```python
from build123d import *

# Parameters (mm, degrees)
BASE_FLANGE1_DEPTH     = 1
SKETCHED_START         = -30
SKETCHED_BEND5_DEPTH   = 60
SKETCHED_BEND5_2_DEPTH = 15
SKETCHED_START_2       = 15
SKETCHED_BEND5_3_DEPTH = 15
SKETCHED_BEND5_4_DEPTH = 60
SKETCHED_START_3       = -15
SKETCHED_BEND5_5_DEPTH = 30
SKETCHED_BEND6_DEPTH   = 60
SKETCHED_BEND6_2_DEPTH = 15
SKETCHED_BEND6_3_DEPTH = 15
SKETCHED_BEND6_4_DEPTH = 30
SKETCHED_BEND6_5_DEPTH = 60
SKETCHED_START_4       = -28.356310605
SKETCHED_BEND7_DEPTH   = 23
SKETCHED_BEND7_2_DEPTH = 23
SKETCHED_START_5       = 11.547743288
SKETCHED_BEND8_DEPTH   = 70
SKETCHED_BEND8_2_DEPTH = 70
SKETCH36_W             = 19.9
SKETCH36_H             = 40.84
CUT_EXTRUDE1_DEPTH     = 10
F_6_CLEARANCE_HOLE4_D  = 3.7973
F_6_CLEARANCE_HOLE2_D  = 3.7973
M1_6_CLEARANCE_HOLE1_D = 1.8
FILLET2_R              = 13
F_2_CLEARANCE_HOLE1_D  = 2.4384
CUT_EXTRUDE2_DEPTH     = 10
FILLET1_R              = 1


# Read off the part's stored shape, not the designer's step: Sketched Bend5, Sketched Bend6, Sketched Bend7, Sketched Bend8
# Sheet-metal steps are written as plain solids
with BuildPart() as part:
    # Sketch1 → Base-Flange1 (new body)
    with BuildSketch(Plane.XY):
        Polygon((-30, -30.5), (-15, -30.5), (-15, -69.5), (15, -69.5), (15, -30.5), (30, -30.5), (30, -7.5), (15, -7.5), (15, 15.5), (30, 15.5), (30, 85.5), (-30, 85.5), (-30, 15.5), (-15, 15.5), (-15, -7.5), (-30, -7.5), align=None)
    extrude(amount=-BASE_FLANGE1_DEPTH)

    # Sketched Bend5 outline → Sketched Bend5 (cut)
    with BuildSketch(Plane.YZ.offset(SKETCHED_START)):
        with BuildLine():
            Line((15.714213562, -0.585786438), (16.128427124, -1))
            Line((16.128427124, -1), (85.5, -1))
            Line((85.5, -1), (85.5, 0))
            Line((85.5, 0), (14.3, 0))
            ThreePointArc((14.3, 0), (15.065366865, -0.152240935), (15.714213562, -0.585786438))
        make_face()
    extrude(amount=SKETCHED_BEND5_DEPTH, mode=Mode.SUBTRACT)

    # Sketched Bend5 2 outline → Sketched Bend5 2 (cut)
    with BuildSketch(Plane.YZ.offset(SKETCHED_START)):
        with BuildLine():
            Line((15.729701149, -0.601274024), (15.714213562, -0.585786438))
            ThreePointArc((15.714213562, -0.585786438), (15.610403483, -0.48909209), (15.5, -0.4))
            Line((15.5, -0.4), (15.5, -0.830975173))
            Line((15.5, -0.830975173), (15.729701149, -0.601274024))
        make_face()
    extrude(amount=SKETCHED_BEND5_2_DEPTH, mode=Mode.SUBTRACT)

    # Sketched Bend5 3 outline → Sketched Bend5 3 (cut)
    with BuildSketch(Plane.YZ.offset(SKETCHED_START_2)):
        with BuildLine():
            Line((15.729701149, -0.601274024), (15.714213562, -0.585786438))
            ThreePointArc((15.714213562, -0.585786438), (15.610403483, -0.48909209), (15.5, -0.4))
            Line((15.5, -0.4), (15.5, -0.830975173))
            Line((15.5, -0.830975173), (15.729701149, -0.601274024))
        make_face()
    extrude(amount=SKETCHED_BEND5_3_DEPTH, mode=Mode.SUBTRACT)

    # Sketched Bend5 4 outline → Sketched Bend5 4 (add)
    with BuildSketch(Plane.YZ.offset(SKETCHED_START)):
        Polygon((65.227175832, -50.098748707), (16.128427124, -1), (15.5, -1), (15.5, -0.830975173), (15.022594368, -1.308380805), (64.520069051, -50.805855488), align=None)
    extrude(amount=SKETCHED_BEND5_4_DEPTH)

    # Sketched Bend5 5 outline → Sketched Bend5 5 (add)
    with BuildSketch(Plane.YZ.offset(SKETCHED_START_3)):
        with BuildLine():
            Line((15.022594368, -1.308380805), (15.330975173, -1))
            Line((15.330975173, -1), (14.3, -1))
            ThreePointArc((14.3, -1), (14.682683432, -1.076120467), (15.007106781, -1.292893219))
            Line((15.007106781, -1.292893219), (15.022594368, -1.308380805))
        make_face()
    extrude(amount=SKETCHED_BEND5_5_DEPTH)

    # Sketched Bend6 outline → Sketched Bend6 (cut)
    with BuildSketch(Plane.YZ.offset(SKETCHED_START)):
        with BuildLine():
            ThreePointArc((-5.710951377, -1), (-6.476318242, -0.847759065), (-7.12516494, -0.414213562))
            Line((-7.12516494, -0.414213562), (-7.539378502, 0))
            Line((-7.539378502, 0), (-69.5, 0))
            Line((-69.5, 0), (-69.5, -1))
            Line((-69.5, -1), (-5.710951377, -1))
        make_face()
    extrude(amount=SKETCHED_BEND6_DEPTH, mode=Mode.SUBTRACT)

    # Sketched Bend6 2 outline → Sketched Bend6 2 (cut)
    with BuildSketch(Plane.YZ.offset(SKETCHED_START)):
        Polygon((-7.539378502, 0), (-7.5, -0.039378502), (-7.5, 0), align=None)
    extrude(amount=SKETCHED_BEND6_2_DEPTH, mode=Mode.SUBTRACT)

    # Sketched Bend6 3 outline → Sketched Bend6 3 (cut)
    with BuildSketch(Plane.YZ.offset(SKETCHED_START_2)):
        Polygon((-7.539378502, 0), (-7.5, -0.039378502), (-7.5, 0), align=None)
    extrude(amount=SKETCHED_BEND6_3_DEPTH, mode=Mode.SUBTRACT)

    # Sketched Bend6 4 outline → Sketched Bend6 4 (add)
    with BuildSketch(Plane.YZ.offset(SKETCHED_START_3)):
        with BuildLine():
            Line((-7.539378502, 0), (-5.710951377, 0))
            ThreePointArc((-5.710951377, 0), (-6.09363481, 0.076120467), (-6.418058159, 0.292893219))
            Line((-6.418058159, 0.292893219), (-50.690686454, 44.565521514))
            Line((-50.690686454, 44.565521514), (-51.397793235, 43.858414733))
            Line((-51.397793235, 43.858414733), (-7.539378502, 0))
        make_face()
    extrude(amount=SKETCHED_BEND6_4_DEPTH)

    # Sketched Bend6 5 outline → Sketched Bend6 5 (add)
    with BuildSketch(Plane.YZ.offset(SKETCHED_START)):
        Polygon((-23.820628769, 16.281250267), (-7.557172802, 0.0177943), (-6.850066021, 0.724901081), (-23.113521988, 16.988357048), align=None)
    extrude(amount=SKETCHED_BEND6_5_DEPTH)

    # Sketched Bend7 outline → Sketched Bend7 (cut)
    with BuildSketch(Plane(origin=(0, 0, 0), x_dir=(1, 0, 0), z_dir=(0, 0.707106781186546, -0.707106781186549)).offset(SKETCHED_START_4)):
        with BuildLine():
            ThreePointArc((-16.732050807, 4.331145665), (-16, 5.063196472), (-15, 5.331145665))
            Line((-15, 5.331145665), (-30, 5.331145665))
            Line((-30, 5.331145665), (-30, 4.331145665))
            Line((-30, 4.331145665), (-16.732050807, 4.331145665))
        make_face()
        with BuildLine():
            Line((30, 5.331145665), (15, 5.331145665))
            ThreePointArc((15, 5.331145665), (16, 5.063196472), (16.732050807, 4.331145665))
            Line((16.732050807, 4.331145665), (30, 4.331145665))
            Line((30, 4.331145665), (30, 5.331145665))
        make_face()
    extrude(amount=SKETCHED_BEND7_DEPTH, mode=Mode.SUBTRACT)

    # Sketched Bend7 2 outline → Sketched Bend7 2 (add)
    with BuildSketch(Plane(origin=(0, 0, 0), x_dir=(1, 0, 0), z_dir=(0, 0.707106781186546, -0.707106781186549)).offset(SKETCHED_START_4)):
        with BuildLine():
            Line((-15, 4.331145665), (-16.732050807, 4.331145665))
            ThreePointArc((-16.732050807, 4.331145665), (-16.931851652, 3.848783755), (-17, 3.331145665))
            Line((-17, 3.331145665), (-17, -9.312659845))
            Line((-17, -9.312659845), (-16, -9.312659845))
            Line((-16, -9.312659845), (-16, 3.331145665))
            ThreePointArc((-16, 3.331145665), (-15.707106781, 4.038252446), (-15, 4.331145665))
        make_face()
        with BuildLine():
            ThreePointArc((17, 3.331145665), (16.931851652, 3.848783755), (16.732050807, 4.331145665))
            Line((16.732050807, 4.331145665), (15, 4.331145665))
            ThreePointArc((15, 4.331145665), (15.707106781, 4.038252446), (16, 3.331145665))
            Line((16, 3.331145665), (16, -9.312659845))
            Line((16, -9.312659845), (17, -9.312659845))
            Line((17, -9.312659845), (17, 3.331145665))
        make_face()
    extrude(amount=SKETCHED_BEND7_2_DEPTH)

    # Sketched Bend8 outline → Sketched Bend8 (cut)
    with BuildSketch(Plane(origin=(0, 0, 0), x_dir=(1, 0, 0), z_dir=(0, 0.707106781186546, -0.707106781186549)).offset(SKETCHED_START_5)):
        with BuildLine():
            Line((-30, -10.697413409), (-16.732050808, -10.697413409))
            ThreePointArc((-16.732050808, -10.697413409), (-16, -9.965362601), (-15, -9.697413409))
            Line((-15, -9.697413409), (-30, -9.697413409))
            Line((-30, -9.697413409), (-30, -10.697413409))
        make_face()
        with BuildLine():
            Line((30, -9.697413409), (15, -9.697413409))
            ThreePointArc((15, -9.697413409), (16, -9.965362601), (16.732050808, -10.697413409))
            Line((16.732050808, -10.697413409), (30, -10.697413409))
            Line((30, -10.697413409), (30, -9.697413409))
        make_face()
    extrude(amount=SKETCHED_BEND8_DEPTH, mode=Mode.SUBTRACT)

    # Sketched Bend8 2 outline → Sketched Bend8 2 (add)
    with BuildSketch(Plane(origin=(0, 0, 0), x_dir=(1, 0, 0), z_dir=(0, 0.707106781186546, -0.707106781186549)).offset(SKETCHED_START_5)):
        with BuildLine():
            ThreePointArc((-16.732050808, -10.697413409), (-16.931851653, -11.179775319), (-17, -11.697413409))
            Line((-17, -11.697413409), (-17, -24.341218918))
            Line((-17, -24.341218918), (-16, -24.341218918))
            Line((-16, -24.341218918), (-16, -11.697413409))
            ThreePointArc((-16, -11.697413409), (-15.707106781, -10.990306628), (-15, -10.697413409))
            Line((-15, -10.697413409), (-16.732050808, -10.697413409))
        make_face()
        with BuildLine():
            Line((16.732050808, -10.697413409), (15, -10.697413409))
            ThreePointArc((15, -10.697413409), (15.707106781, -10.990306628), (16, -11.697413409))
            Line((16, -11.697413409), (16, -24.341218918))
            Line((16, -24.341218918), (17, -24.341218918))
            Line((17, -24.341218918), (17, -11.697413409))
            ThreePointArc((17, -11.697413409), (16.931851653, -11.179775319), (16.732050808, -10.697413409))
        make_face()
    extrude(amount=SKETCHED_BEND8_2_DEPTH)

    # Sketch36 → Cut-Extrude1 (cut)
    with BuildSketch(Plane(origin=(0, 7.564213562, 7.564213562), x_dir=(1, 0, 0), z_dir=(0, 0.7071067811865487, 0.7071067811865465))):
        with Locations((0, 51.627743288)):
            Rectangle(SKETCH36_W, SKETCH36_H)
    extrude(amount=-CUT_EXTRUDE1_DEPTH, mode=Mode.SUBTRACT)

    # #6 Clearance Hole4 (through all)
    with Locations(Plane(origin=(0, 7.564213562, 7.564213562), x_dir=(1, 0, 0), z_dir=(0, 0.7071067811865487, 0.7071067811865465))):
        with Locations((-4.97, 76.727743288), (4.97, 76.727743288), (-4.97, 26.527743288), (4.97, 26.527743288), (-8.5, 18.025840533), (8.5, 18.025840533), (0, -14.745359227), (-8.5, -36.745359227), (8.5, -36.745359227)):
            Hole(F_6_CLEARANCE_HOLE4_D / 2)

    # #6 Clearance Hole2 (through all)
    with Locations(Plane(origin=(17, 0, 0), x_dir=(0, 0, -1), z_dir=(1, 0, 0))):
        with Locations((-9.311868306, -5.334166607), (-16.382936118, -12.405234419), (-0.914625389, 24.316668374), (6.156442422, 31.387736186)):
            Hole(F_6_CLEARANCE_HOLE2_D / 2)

    # M1.6 Clearance Hole1 (through all)
    with Locations(Plane(origin=(0, -3.06258247, -3.06258247), x_dir=(1, 0, 0), z_dir=(0, 0.7071067811865487, 0.7071067811865465))):
        with Locations((0, -47.221310605), (-3.48, -47.221310605), (3.48, -47.221310605), (-3.48, -62.491310605), (0, -62.491310605), (3.48, -62.491310605), (7.635, -58.336310605), (7.635, -54.856310605), (7.635, -51.376310605), (-7.635, -58.336310605), (-7.635, -54.856310605), (-7.635, -51.376310605)):
            Hole(M1_6_CLEARANCE_HOLE1_D / 2)

    # Fillet2
    fillet2_edges = [part.edges().sort_by_distance(p)[0] for p in [
        (-15, -51.044239844, 44.211968124),
        (15, -51.044239844, 44.211968124),
    ]]
    fillet(fillet2_edges, radius=FILLET2_R)

    # #2 Clearance Hole1 (through all)
    with Locations(Plane(origin=(0, -3.769689251, -3.769689251), x_dir=(-1, 0, 0), z_dir=(0, -0.7071067811865487, -0.7071067811865465))):
        with Locations((0, -54.856310605)):
            Hole(F_2_CLEARANCE_HOLE1_D / 2)

    # Sketch51 → Cut-Extrude2 (cut)
    with BuildSketch(Plane.XY):
        Polygon((-10, 10.8), (10, 10.8), (5, 5.8), (-5, 5.8), align=None)
        Polygon((-5, 2.789048623), (5, 2.789048623), (10, -2.210951377), (-10, -2.210951377), align=None)
    extrude(amount=-CUT_EXTRUDE2_DEPTH, mode=Mode.SUBTRACT)

    # Fillet1
    fillet1_edges = [part.edges().sort_by_distance(p)[0] for p in [
        (-16.5, -13.465894591, 26.635984446),
        (-16.5, 2.797561376, 10.372528478),
        (16.5, 2.797561376, 10.372528478),
        (16.5, -13.465894591, 26.635984446),
        (-16.5, 25.377328546, 9.046353373),
        (-16.5, 74.874803229, -40.45112131),
        (16.5, 74.874803229, -40.45112131),
        (16.5, 25.377328546, 9.046353373),
        (-5, 5.8, -0.5),
        (-10, 10.8, -0.5),
        (10, 10.8, -0.5),
        (5, 5.8, -0.5),
        (-10, -2.210951377, -0.5),
        (-5, 2.789048623, -0.5),
        (5, 2.789048623, -0.5),
        (10, -2.210951377, -0.5),
    ]]
    fillet(fillet1_edges, radius=FILLET1_R)


solid = part.part
```
Verification items for the finished model (mm, model axes). A direction names the side the tool comes from. Coordinates: 2 decimals unless noted, no trailing zeros. Return JSON: item names as keys, results as strings.
1. Thickness scan on L1, parallel to X at y = 69.5, z = -45; L2, parallel to Z at x = 8, y = -3; L3, parallel to Z at x = -4.5, y = -42. Record the ranges inside material, lowest first.
Established:
{"L1": "x = -17 to -16, 16 to 17", "L2": "z = -1 to 0", "L3": "z = 34.46 to 35.87"}
2. Tool access check on faces 1 (the cylindrical face through (15.7, 40.33, -24.8)), 2 (the cylindrical face through (10.397, 20.011, -5.6)), 3 (the flat face through (-16.5, -19.1, 21)), 4 (the flat face through (-6.8, 7.6, -0.5)), 5 (the flat face through (-16.46, 19.78, 3.45)). Record the directions out of +Z, -Z, +X, -X, +Y, -Y that give a thin tool (end or side, any length) a straight path to the whole face; none if there is none.
Established:
{"face 1": "+Z, +Y", "face 2": "none", "face 3": "+Z, -X, -Y", "face 4": "+Z, -Z", "face 5": "+Z, -X"}
3. Go/stop test with flat-tipped pins: pin 1 (3.5 mm diameter, centred on y = -12.41, z = 16.38, fed in from +X); pin 2 (1.5 mm diameter, centred on x = 13.5, z = 34.5, fed in from +Y); pin 3 (3 mm diameter, centred on x = -1.5, y = 21, fed in from +Z); pin 4 (10 mm diameter, centred on x = 0.5, y = 2.5, fed in from +Z). Record where each tip stops, or that it passes through.
Established:
{"pin 1": "passes through", "pin 2": "stops at y = -39.88", "pin 3": "stops at z = -4.37", "pin 4": "stops at z = 0"}
4. Mould release check, pull along X, two halves, no side actions. Record for faces 6 (the cylindrical face through (-16.507, -7.188, 8.9)), 7 (the cylindrical face through (5.217, 27.295, -12.883)), 8 (the flat face through (15, -32, 25)): +X half, -X half, draft (parallel to the pull), parting line (faces both ways), or undercut.
Established:
{"face 6": "draft", "face 7": "undercut", "face 8": "+X half"}
